Autodesk Inventor part; units mm, degrees
ref_plane "Work Plane1" through (0, 15, 0) normal (0, 1, 0) x (1, 0, 0)
ref_plane "Work Plane2" through (0, 10, 0) normal (0, 1, 0) x (1, 0, 0)
ref_plane "YZ Plane" through (0, 0, 0) normal (1, 0, 0) x (0, 1, 0)
sketch "Sketch1" plane through (0, 0, 0) normal (0, 1, 0) x (-1, 0, 0)
  circle A0 centre (0, 0) radius 4.3656
  dimension "d0" = 8.7312
extrude "Extrusion1" add sketch "Sketch1" along normal blind 10
thread "Thread1"
sketch "Sketch2" plane through (0, 10, 0) normal (0, 1, 0) x (1, 0, 0)
  circle A0 centre (0, 0) radius 5
  dimension "d5" = 10
ref_plane "Work Plane1" through (0, 15, 0) normal (0, 1, 0) x (1, 0, 0)
sketch "Sketch3" plane through (0, 15, 0) normal (0, 1, 0) x (1, 0, 0)
  circle A0 centre (0, 0) radius 4
  dimension "d7" = 8
loft "Loft1" add profiles "Sketch2", "Sketch3"
sketch "Sketch4" plane through (0, 15, 0) normal (0, 1, 0) x (1, 0, 0)
  circle A0 centre (0, 0) radius 3.5
  dimension "d12" = 7
ref_plane "Work Plane2" through (0, 10, 0) normal (0, 1, 0) x (1, 0, 0)
sketch "Sketch5" plane through (0, 10, 0) normal (0, 1, 0) x (1, 0, 0)
  circle A0 centre (0, 0) radius 2.5
  dimension "d14" = 5
loft "Loft2" cut profiles "Sketch5", "Sketch4"
sketch "Sketch6" plane through (0, 10, 0) normal (0, 1, 0) x (1, 0, 0)
  circle A0 centre (0, 0) radius 2.4663
extrude "Extrusion2" add sketch "Sketch6" along normal blind 3
fillet "Fillet1" radius 2.4 1 edges at (-2.4663, 13, 0)
properties part number "LED Holder"
The model under review builds one solid part; all positions refer to its coordinate system, in mm. Round coordinates to 2 decimals unless told otherwise and drop trailing zeros. Loops run counter-clockwise (first coordinate to the right, second up) from the corner with the lowest first, then second, coordinate; pieces in that order, holes last. Notation, with made-up numbers: (-14.5, 32.5) - (42.5, 32.5) arc R26 cw to (42.5, 52.5) - close; hole circle Ø11 at (23.5, 67). An arc over 180 degrees is marked (long way). Use a Markdown table: item, result. Add a question column.
Q1. Add section B-B (y = 3.25). State the section outline as (x, z) points, plus the area to 3 significant figures.
Q2. Add section C-C (y = 12.25). State how many separate pieces and enclosed holes the cut face has, plus the area to 3 significant figures.
Q3. The part is to be moulded in two halves that separate along Z. For faces 1 (the face through (-0.38, 11.98, -2.87)), 2 (the face through (0.57, 4.93, -4.33)), 3 (the face through (2.6, 10, 3.7)), say which applies: pulls with the +Z half, pulls with the -Z half, needs draft (parallel to the pull), parting line crosses it, or undercut.
Q4. Add section A-A (y = 10.25). State the section outline as (x, z) points, plus the area to 3 significant figures.
Q5. For probe 1 along Z at (x, y) = (0, 11.75); probe 2 along X at (y, z) = (13.5, 1.75); probe 3 along Z at (x, y) = (3, 8.25), list the stretches that pass through material, from the lowest coordinate up.
Q6. Insertion check: pin 1 Ø6 at (x, z) = (-1, -2.5) entering from -Y; pin 2 Ø1 at (x, y) = (2, 11.5) entering from +Z; pin 3 Ø5 at (y, z) = (4, 0.5) entering from +X; pin 4 Ø4 at (x, y) = (1, 12.5) entering from -Z. Each pin has a flat end and moves straight along its axis. Give the tip position at first contact, or say it passes through.
Worked answers:
| question | item | result |
|---|---|---|
| 1 | outline | circle Ø8.73 at (0, 0) |
| 1 | area | 59.9 mm² |
| 2 | separate pieces | 2 |
| 2 | enclosed holes | 1 |
| 2 | area | 48.0 mm² |
| 3 | face 1 | undercut |
| 3 | face 2 | parting line crosses it |
| 3 | face 3 | needs draft |
| 4 | outline | circle Ø9.9 at (0, 0); circle Ø4.93 at (0, 0); hole circle Ø5.1 at (0, 0) |
| 4 | area | 75.7 mm² |
| 5 | probe 1 | -4.65 to -2.85, -2.17 to 2.17, 2.85 to 4.65 |
| 5 | probe 2 | -3.93 to -2.68, 2.68 to 3.93 |
| 5 | probe 3 | -3.17 to 3.17 |
| 6 | pin 1 | y = 0 |
| 6 | pin 2 | z = 4.48 |
| 6 | pin 3 | x = 4.37 |
| 6 | pin 4 | z = -4.87 |
